Geometry check sheet. Reference: the model listing, model coordinates, mm. Coordinates: 2 decimals unless noted, no trailing zeros. Write each loop counter-clockwise with the first axis right and the second up, starting at its lowest first coordinate (ties: lowest second). Pieces come first, ordered by that corner, then holes. Notation, with made-up numbers: (52, 7.25) -> (103, 7.25) arc R26 ccw to (103, 43.25) -> close; hole circle Ø6 at (73.5, 57.25). An arc over 180 degrees is marked (long way). Use a Markdown table: item, result.
```python
from build123d import *

# Parameters (mm, degrees)
SKETCH_1_R          = 8.4
EXTRUDE_1_DEPTH     = 7.5
SKETCH_2_R          = 3.3
CUT_EXTRUDE_1_DEPTH = 15
FILLET_1_R          = 2


with BuildPart() as part:
    # 草图1 → 凸台-拉伸1 (new, symmetric)
    with BuildSketch(Plane(origin=(0, 0, 0), x_dir=(0, 0, -1), z_dir=(1, 0, 0))):
        Circle(SKETCH_1_R)
    extrude(amount=EXTRUDE_1_DEPTH, both=True)

    # 草图2 → 切除-拉伸1 (cut)
    with BuildSketch(Plane(origin=(7.5, 0, 0), x_dir=(0, 0, -1), z_dir=(1, 0, 0))):
        Circle(SKETCH_2_R)
    extrude(amount=-CUT_EXTRUDE_1_DEPTH, mode=Mode.SUBTRACT)

    # 圆角1
    fillet_1_edges = [part.edges().sort_by_distance(p)[0] for p in [
        (-7.5, 0, 8.4),
        (7.5, 0, 8.4),
    ]]
    fillet(fillet_1_edges, radius=FILLET_1_R)


solid = part.part
```
Item 1: Depth check by flat-ended pin: P1, Ø3, axis at x = 3.5, z = -2, coming from the +Y side; P2, Ø4, axis at y = 0, z = 0, coming from the -X side; P3, Ø1.5, axis at x = -5, y = -6, coming from the -Z side; P4, Ø3, axis at x = 0.5, z = 2.5, coming from the -Y side. Enter the tip coordinate at first touch or a pass-through.
Answer block:
| item | result |
|---|---|
| P1 | stops at y = 8.39 |
| P2 | passes through |
| P3 | stops at z = -6.56 |
| P4 | stops at y = -8.34 |
Item 2: Section check C-C on x = -2. Record the boundary of the cut face in (y, z).
Answer block:
| item | result |
|---|---|
| outline | circle Ø16.8 at (0, 0); hole circle Ø6.6 at (0, 0) |
Item 3: Thickness scan on L1, parallel to Y at x = 3.5, z = 0; L2, parallel to Z at x = -3.75, y = -0.75; L3, parallel to X at y = -6, z = -2.5. Record the ranges inside material, lowest first. Write a range as [from, to].
Answer block:
| item | result |
|---|---|
| L1 | y = [-8.4, -3.3], [3.3, 8.4] |
| L2 | z = [-8.37, -3.21], [3.21, 8.37] |
| L3 | x = [-7.5, 7.5] |
Item 4: Mould release check, pull along Y, two halves, no side actions. Record for faces 1 (the cylindrical face through (0.077, 2.523, -8.012)), 2 (the cylindrical face through (0.11, 2.23, 2.43)), 3 (the flat face through (7.5, 2, 3)): +Y half, -Y half, draft (parallel to the pull), parting line (faces both ways), or undercut.
Answer block:
| item | result |
|---|---|
| face 1 | parting line |
| face 2 | undercut |
| face 3 | draft |
Item 5: Section check A-A on y = 0. Record the boundary of the cut face in (x, z), then the cut area to 3 significant figures.
Answer block:
| item | result |
|---|---|
| outline | (-7.5, -6.4) arc R2 ccw to (-5.5, -8.4) -> (5.5, -8.4) arc R2 ccw to (7.5, -6.4) -> (7.5, -3.3) -> (-7.5, -3.3) -> close; (-7.5, 3.3) -> (7.5, 3.3) -> (7.5, 6.4) arc R2 ccw to (5.5, 8.4) -> (-5.5, 8.4) arc R2 ccw to (-7.5, 6.4) -> close |
| area | 150 mm^2 |
